from build123d import *

# Parameters (mm, degrees)
ESBO_O1_R                     = 35
ESBO_O1_R_2                   = 32.5
RESSALTO_EXTRUS_O1_DEPTH      = 8
RESSALTO_EXTRUS_O2_START      = -3
ESBO_O2_R                     = 32.5
RESSALTO_EXTRUS_O2_DEPTH      = 3
ESBO_O3_R                     = 2.5
CORTE_EXTRUS_O1_DEPTH         = 3
RESSALTO_EXTRUS_O3_DEPTH      = 5
RESSALTO_EXTRUS_O3_DEPTH_BACK = 3
ESBO_O4_R                     = 37
ESBO_O4_R_2                   = 35
ESBO_O5_W                     = 1.8
ESBO_O5_H                     = 3
ESBO_O6_R                     = 12.55
RESSALTO_EXTRUS_O4_DEPTH      = 5
CORTE_EXTRUS_O2_DEPTH         = 53.933921071
CORTE_EXTRUS_O2_DEPTH_BACK    = 53.933921071
ESBO_O7_R                     = 7.55
RESSALTO_EXTRUS_O5_START      = -8
ESBO_O8_R                     = 37
ESBO_O8_R_2                   = 32.5
RESSALTO_EXTRUS_O5_DEPTH      = 8
ESBO_O9_R                     = 37
ESBO_O9_R_2                   = 33.5
CORTE_EXTRUS_O8_DEPTH         = 1.5
CORTE_EXTRUS_O9_START         = -1.5
ESBO_O12_R                    = 37
ESBO_O12_R_2                  = 33.5
CORTE_EXTRUS_O9_DEPTH         = 1.5
CORTE_EXTRUS_O10_START        = -10
ESBO_O13_R                    = 37
ESBO_O13_R_2                  = 36
CORTE_EXTRUS_O10_DEPTH        = 10
ESBO_O14_R                    = 37
ESBO_O14_R_2                  = 36
RESSALTO_EXTRUS_O6_DEPTH      = 5
ESBO_O15_R                    = 12.55
CORTE_EXTRUS_O11_DEPTH        = 53.933921071
ESBO_O16_R                    = 12.55
RESSALTO_EXTRUS_O7_DEPTH      = 3
ESBO_O17_R                    = 10
RESSALTO_EXTRUS_O8_DEPTH      = 16
ESBO_O18_R                    = 3.3
CORTE_EXTRUS_O12_DEPTH        = 16
ESBO_O19_W                    = 5.95
ESBO_O19_H                    = 2.65
CORTE_EXTRUS_O13_DEPTH        = 8
CORTE_EXTRUS_O14_DEPTH        = 58.265085349
CORTE_EXTRUS_O14_DEPTH_BACK   = 58.265085349
ESBO_O21_R                    = 1.65
ESBO_O23_R                    = 37
ESBO_O23_R_2                  = 36
CORTE_EXTRUS_O15_DEPTH        = 54.798234195


with BuildPart() as part:
    # Esboço1 → Ressalto-extrusão1 (new body)
    with BuildSketch(Plane.XY):
        Circle(ESBO_O1_R)
        Circle(ESBO_O1_R_2, mode=Mode.SUBTRACT)
    extrude(amount=RESSALTO_EXTRUS_O1_DEPTH)

    # Esboço2 → Ressalto-extrusão2 (add)
    with BuildSketch(Plane.XY.offset(8).offset(RESSALTO_EXTRUS_O2_START)):
        Circle(ESBO_O2_R)
    extrude(amount=RESSALTO_EXTRUS_O2_DEPTH)

    # Esboço3 → Corte-extrusão1 (cut)
    with BuildSketch(Plane.XY.offset(8)):
        Circle(ESBO_O3_R)
    extrude(amount=-CORTE_EXTRUS_O1_DEPTH, mode=Mode.SUBTRACT)

    # Esboço4 → Ressalto-extrusão3 (add, two sides: drawn at the far end of the back side and taken through both)
    with BuildSketch(Plane(origin=(0, 0, 5), x_dir=(-1, 0, 0), z_dir=(0, 0, -1)).offset(-RESSALTO_EXTRUS_O3_DEPTH_BACK)):
        Circle(ESBO_O4_R)
        Circle(ESBO_O4_R_2, mode=Mode.SUBTRACT)
    extrude(amount=RESSALTO_EXTRUS_O3_DEPTH + RESSALTO_EXTRUS_O3_DEPTH_BACK)

    # Esboço5 → Corte-Revolução1 (revolve, cut)
    with BuildSketch(Plane(origin=(0, 0, 0), x_dir=(1, 0, 0), z_dir=(0, 1, 0))):
        with Locations((-36.1, -2.5)):
            Rectangle(ESBO_O5_W, ESBO_O5_H)
        with Locations((-36.1, -5.5)):
            Rectangle(ESBO_O5_W, ESBO_O5_H)
    revolve(axis=Axis((0, 0, 8), (0, 0, -1)), mode=Mode.SUBTRACT)

    # Esboço6 → Ressalto-extrusão4 (add)
    with BuildSketch(Plane(origin=(0, 0, 5), x_dir=(-1, 0, 0), z_dir=(0, 0, -1))):
        with Locations(Location((0, 0, 0), (0, 0, 180))):
            Circle(ESBO_O6_R)
    extrude(amount=RESSALTO_EXTRUS_O4_DEPTH)

    # Esboço7 → Corte-extrusão2 (cut, two sides: drawn at the far end of the back side and taken through both)
    with BuildSketch(Plane(origin=(0, 0, 0), x_dir=(-1, 0, 0), z_dir=(0, 0, -1)).offset(-CORTE_EXTRUS_O2_DEPTH_BACK)):
        Circle(ESBO_O7_R)
    extrude(amount=CORTE_EXTRUS_O2_DEPTH + CORTE_EXTRUS_O2_DEPTH_BACK, mode=Mode.SUBTRACT)

    # Esboço8 → Ressalto-extrusão5 (add)
    with BuildSketch(Plane.XY.offset(8).offset(RESSALTO_EXTRUS_O5_START)):
        with Locations(Location((0, 0, 0), (0, 0, 180))):
            Circle(ESBO_O8_R)
        Circle(ESBO_O8_R_2, mode=Mode.SUBTRACT)
    extrude(amount=RESSALTO_EXTRUS_O5_DEPTH)

    # Esboço9 → Corte-extrusão8 (cut)
    with BuildSketch(Plane.XY.offset(8)):
        with Locations(Location((0, 0, 0), (0, 0, 180))):
            Circle(ESBO_O9_R)
        Circle(ESBO_O9_R_2, mode=Mode.SUBTRACT)
    extrude(amount=-CORTE_EXTRUS_O8_DEPTH, mode=Mode.SUBTRACT)

    # Esboço12 → Corte-extrusão9 (cut)
    with BuildSketch(Plane(origin=(0, 0, 0), x_dir=(-1, 0, 0), z_dir=(0, 0, -1)).offset(CORTE_EXTRUS_O9_START)):
        Circle(ESBO_O12_R)
        with Locations(Location((0, 0, 0), (0, 0, 180))):
            Circle(ESBO_O12_R_2, mode=Mode.SUBTRACT)
    extrude(amount=CORTE_EXTRUS_O9_DEPTH, mode=Mode.SUBTRACT)

    # Esboço13 → Corte-extrusão10 (cut)
    with BuildSketch(Plane(origin=(0, 0, 1.5), x_dir=(-1, 0, 0), z_dir=(0, 0, -1)).offset(CORTE_EXTRUS_O10_START)):
        Circle(ESBO_O13_R)
        Circle(ESBO_O13_R_2, mode=Mode.SUBTRACT)
    extrude(amount=CORTE_EXTRUS_O10_DEPTH, mode=Mode.SUBTRACT)

    # Esboço14 → Ressalto-extrusão6 (add)
    with BuildSketch(Plane.XY.offset(6.5)):
        Circle(ESBO_O14_R)
        Circle(ESBO_O14_R_2, mode=Mode.SUBTRACT)
    extrude(amount=-RESSALTO_EXTRUS_O6_DEPTH)

    # Esboço15 → Corte-extrusão11 (cut, through all)
    with BuildSketch(Plane(origin=(0, 0, 0), x_dir=(-1, 0, 0), z_dir=(0, 0, -1))):
        Circle(ESBO_O15_R)
    extrude(amount=-CORTE_EXTRUS_O11_DEPTH, mode=Mode.SUBTRACT)

    # Esboço16 → Ressalto-extrusão7 (add, through all)
    with BuildSketch(Plane(origin=(0, 0, 5), x_dir=(-1, 0, 0), z_dir=(0, 0, -1))):
        Circle(ESBO_O16_R)
    extrude(amount=-RESSALTO_EXTRUS_O7_DEPTH)

    # Esboço17 → Ressalto-extrusão8 (add)
    with BuildSketch(Plane(origin=(0, 0, 5), x_dir=(-1, 0, 0), z_dir=(0, 0, -1))):
        with Locations(Location((0, 0, 0), (0, 0, 180))):
            Circle(ESBO_O17_R)
    extrude(amount=RESSALTO_EXTRUS_O8_DEPTH)

    # Esboço18 → Corte-extrusão12 (cut)
    with BuildSketch(Plane(origin=(0, 0, -11), x_dir=(-1, 0, 0), z_dir=(0, 0, -1))):
        Circle(ESBO_O18_R)
    extrude(amount=-CORTE_EXTRUS_O12_DEPTH, mode=Mode.SUBTRACT)

    # Esboço19 → Corte-extrusão13 (cut)
    with BuildSketch(Plane(origin=(0, 0, -11), x_dir=(-1, 0, 0), z_dir=(0, 0, -1))):
        with Locations((0, -6.625)):
            Rectangle(ESBO_O19_W, ESBO_O19_H)
        with Locations((0, 6.625)):
            Rectangle(ESBO_O19_W, ESBO_O19_H)
    extrude(amount=-CORTE_EXTRUS_O13_DEPTH, mode=Mode.SUBTRACT)

    # Esboço21 → Corte-extrusão14 (cut, two sides: drawn at the far end of the back side and taken through both)
    with BuildSketch(Plane(origin=(0, 5.3, 0), x_dir=(1, 0, 0), z_dir=(0, 1, 0)).offset(-CORTE_EXTRUS_O14_DEPTH_BACK)):
        with Locations(Location((0, 6.85, 0), (0, 0, 180))):
            Circle(ESBO_O21_R)
    extrude(amount=CORTE_EXTRUS_O14_DEPTH + CORTE_EXTRUS_O14_DEPTH_BACK, mode=Mode.SUBTRACT)

    # Esboço23 → Corte-extrusão15 (cut, through all)
    with BuildSketch(Plane(origin=(0, 0, 1.5), x_dir=(-1, 0, 0), z_dir=(0, 0, -1))):
        Circle(ESBO_O23_R)
        Circle(ESBO_O23_R_2, mode=Mode.SUBTRACT)
    extrude(amount=-CORTE_EXTRUS_O15_DEPTH, mode=Mode.SUBTRACT)


solid = part.part
Work out the finished part from the listing and answer in its coordinate system (mm). A direction names the side the tool comes from. Coordinates: 2 decimals unless noted, no trailing zeros. Order: outer loops, then holes, each group sorted by start corner. A loop starts at its lowest first (then second) coordinate and runs counter-clockwise, first axis right, second up. Notation, with made-up numbers: (78, -21.5) - (110, -21.5) arc R27 ccw to (110, 3.5) - close; hole circle Ø10 at (26, -6). An arc over 180 degrees is marked (long way). Put each result on its own line as item: value. Start each with the question number.
1) For faces 4 (the cylindrical face through (-2.17, 9.76, -2.89)), 5 (the flat face through (4, 0, -11)), determine the directions among +Z, -Z, +X, -X, +Y, -Y from which every point of the face is accessible in a straight line to the end or side of a thin tool.
2) For a pull along Z with two mould halves and no side action, classify faces 1 (the cylindrical face through (-0.761, -4.096, -8.314)), 2 (the flat face through (-2.975, -7, -7)), 3 (the flat face through (0, 7, -3)) as released by +Z, released by -Z, zero draft, split by the parting line, or undercut.
3) Find section A-A (z = -6.85). Give the vertices of the cut face in (x, y) (3 decimals).
4) Find section C-C (x = 12). Give the vertices of the cut face in (y, z).
5) Flat-ended cylindrical pins translate along their axes: pin 1 (0.8 mm diameter, centred on y = -6.5, z = -9, fed in from -X); pin 2 (5 mm diameter, centred on x = -25, z = -2, fed in from +Y); pin 3 (6 mm diameter, centred on y = -10.5, z = -6.5, fed in from +X). Find the tip coordinate at first contact, or state that the pin passes through.
6) Find section D-D (x = 0). State how many separate pieces and enclosed holes the cut face has, plus the area to 3 significant figures.
7) Find the intervals of material crossed by line 1 (Y direction, x = 0, z = 2.35); line 2 (Y direction, x = 2, z = -6); line 3 (Z direction, x = 0, y = 4.65), in increasing order. Write a range as from..to.
8) Find section B-B (y = 0). Give the vertices of the cut face in (x, z), plus the area to 3 significant figures.
Results list:
1. face 4: -Z
1. face 5: -Z, +X, -X, +Y, -Y
2. face 1: undercut
2. face 2: zero draft
2. face 3: released by -Z
3. outline: (-2.975, -7.95) - (-2.975, -5.3) - (-1.65, -5.3) - (-1.65, -2.858) arc R3.3 cw to (-1.65, 2.858) - (-1.65, 5.3) - (-2.975, 5.3) - (-2.975, 7.95) - (-1.65, 7.95) - (-1.65, 9.863) arc R10 ccw to (-1.65, -9.863) - (-1.65, -7.95) - close; (1.65, -9.863) arc R10 ccw to (1.65, 9.863) - (1.65, 7.95) - (2.975, 7.95) - (2.975, 5.3) - (1.65, 5.3) - (1.65, 2.858) arc R3.3 cw to (1.65, -2.858) - (1.65, -5.3) - (2.975, -5.3) - (2.975, -7.95) - (1.65, -7.95) - close
4. outline: (-33.94, 1.5) - (-31.28, 1.5) - (-31.28, 0) - (-30.2, 0) - (-30.2, 5) - (30.2, 5) - (30.2, 0) - (31.28, 0) - (31.28, 1.5) - (33.94, 1.5) - (33.94, 6.5) - (31.28, 6.5) - (31.28, 8) - (-31.28, 8) - (-31.28, 6.5) - (-33.94, 6.5) - close
5. pin 1: stops at x = -7.92
5. pin 2: stops at y = 23.87
5. pin 3: stops at x = 6.61
6. separate pieces: 5
6. enclosed holes: 0
6. area: 381 mm^2
7. line 1: y = -36..-32.5, -10..-3.3, 3.3..10, 32.5..36
7. line 2: y = -9.8..-7.95, -5.3..-2.62, 2.62..5.3, 7.95..9.8
7. line 3: z = -11..-8.5, -5.2..8
8. outline: (-36, 1.5) - (-33.5, 1.5) - (-33.5, 0) - (-32.5, 0) - (-32.5, 5) - (-10, 5) - (-10, -11) - (-3.3, -11) - (-3.3, 5) - (3.3, 5) - (3.3, -11) - (10, -11) - (10, 5) - (32.5, 5) - (32.5, 0) - (33.5, 0) - (33.5, 1.5) - (36, 1.5) - (36, 6.5) - (33.5, 6.5) - (33.5, 8) - (-33.5, 8) - (-33.5, 6.5) - (-36, 6.5) - close
8. area: 450 mm^2
